Build history of the part. All positions in model axes, mm. A direction names the side the tool comes from. Coordinates: 2 decimals unless noted, no trailing zeros. Order: outer loops, then holes, each group sorted by start corner. A loop starts at its lowest first (then second) coordinate and runs counter-clockwise, first axis right, second up. Notation, with made-up numbers: (31.25, 46.25) -> (61.25, 46.25) arc R13 cw to (61.25, 62.25) -> close; hole circle Ø8 at (73, 24.5). An arc over 180 degrees is marked (long way). Write each question's results on one line, items separated by ' | '.
from build123d import *

# Parameters (mm, degrees)
SKETCH1_W           = 3
SKETCH1_H           = 3
BOSS_EXTRUDE1_DEPTH = 4
SKETCH2_W           = 19
SKETCH2_H           = 19
BOSS_EXTRUDE2_DEPTH = 6
SKETCH3_R           = 13
BOSS_EXTRUDE3_DEPTH = 4
SKETCH4_R           = 7
BOSS_EXTRUDE4_DEPTH = 10
SKETCH5_R           = 12
BOSS_EXTRUDE5_DEPTH = 4
SKETCH6_R           = 5
CUT_EXTRUDE1_DEPTH  = 6


with BuildPart() as part:
    # Sketch1 → Boss-Extrude1 (new body)
    with BuildSketch(Plane(origin=(0, 0, 0), x_dir=(0, 0, -1), z_dir=(1, 0, 0))):
        Rectangle(SKETCH1_W, SKETCH1_H)
    extrude(amount=BOSS_EXTRUDE1_DEPTH)

    # Sketch2 → Boss-Extrude2 (add)
    with BuildSketch(Plane(origin=(4, 0, 0), x_dir=(0, 0, -1), z_dir=(1, 0, 0))):
        Rectangle(SKETCH2_W, SKETCH2_H)
    extrude(amount=BOSS_EXTRUDE2_DEPTH)

    # Sketch3 → Boss-Extrude3 (add)
    with BuildSketch(Plane(origin=(10, 0, 0), x_dir=(0, 0, -1), z_dir=(1, 0, 0))):
        Circle(SKETCH3_R)
    extrude(amount=BOSS_EXTRUDE3_DEPTH)

    # Sketch4 → Boss-Extrude4 (add)
    with BuildSketch(Plane(origin=(14, 0, 0), x_dir=(0, 0, -1), z_dir=(1, 0, 0))):
        Circle(SKETCH4_R)
    extrude(amount=BOSS_EXTRUDE4_DEPTH)

    # Sketch5 → Boss-Extrude5 (add)
    with BuildSketch(Plane(origin=(24, 0, 0), x_dir=(0, 0, -1), z_dir=(1, 0, 0))):
        Circle(SKETCH5_R)
    extrude(amount=BOSS_EXTRUDE5_DEPTH)

    # Sketch6 → Cut-Extrude1 (cut)
    with BuildSketch(Plane(origin=(28, 0, 0), x_dir=(0, 0, -1), z_dir=(1, 0, 0))):
        Circle(SKETCH6_R)
    extrude(amount=-CUT_EXTRUDE1_DEPTH, mode=Mode.SUBTRACT)


solid = part.part
Item 1: Tool access for faces 1 (the flat face through (2, 0, 1.5)), 2 (the cylindrical face through (25.97, 0.53, 11.99)), 3 (the flat face through (2, 1.5, 0)): list every direction of +Z, -Z, +X, -X, +Y, -Y with a clear straight run to the whole face (end or side of a thin tool).
Answer:
face 1: +Z, -X, +Y, -Y | face 2: +X | face 3: +Z, -Z, -X, +Y
Item 2: Pin check, flat tips, straight feed: pin 1 (8 mm diameter, centred on x = 5, z = 1.5, fed in from +Y); pin 2 (4 mm diameter, centred on y = -4, z = -10.5, fed in from -X); pin 3 (1 mm diameter, centred on x = 10, y = 7, fed in from -Z). Stop position of each tip, or through.
Answer:
pin 1: stops at y = 9.5 | pin 2: stops at x = 4 | pin 3: stops at z = -11.26
Item 3: Slice it at A-A, the plane y = 0. List the corners of the cut face in (x, z), and give its area (3 significant figures).
Answer:
outline: (0, -1.5) -> (4, -1.5) -> (4, -9.5) -> (10, -9.5) -> (10, -13) -> (14, -13) -> (14, -7) -> (24, -7) -> (24, -12) -> (28, -12) -> (28, -5) -> (22, -5) -> (22, 5) -> (28, 5) -> (28, 12) -> (24, 12) -> (24, 7) -> (14, 7) -> (14, 13) -> (10, 13) -> (10, 9.5) -> (4, 9.5) -> (4, 1.5) -> (0, 1.5) -> close | area: 406 mm^2
Item 4: Slice it at C-C, the plane x = 19. List the corners of the cut face in (y, z), and give its area (3 significant figures).
Answer:
outline: circle Ø14 at (0, 0) | area: 154 mm^2
Item 5: Pull direction X, two halves, no side cores. Call faces 4 (the flat face through (22, 0, 0)), 5 (the flat face through (24, -5.2, -5.2)), 6 (the flat face through (7, 9.5, 0)): released by +X, released by -X, zero draft, split by the parting line, or undercut.
Answer:
face 4: released by +X | face 5: undercut | face 6: zero draft
Item 6: Slice it at D-D, the plane z = 6. List the corners of the cut face in (x, y), and give its area (3 significant figures).
Answer:
outline: (4, -9.5) -> (10, -9.5) -> (10, -11.53) -> (14, -11.53) -> (14, -3.61) -> (24, -3.61) -> (24, -10.39) -> (28, -10.39) -> (28, 10.39) -> (24, 10.39) -> (24, 3.61) -> (14, 3.61) -> (14, 11.53) -> (10, 11.53) -> (10, 9.5) -> (4, 9.5) -> close | area: 362 mm^2
Item 7: Drill centre lines: line 1 (X direction, y = 7.25, z = 5.25); line 2 (X direction, y = 11, z = -2.5); line 3 (Y direction, x = 23.75, z = 0). Where is each one in solid material? Low to high. Write a range as from..to.
Answer:
line 1: x = 4..14, 24..28 | line 2: x = 10..14, 24..28 | line 3: y = -7..-5, 5..7
